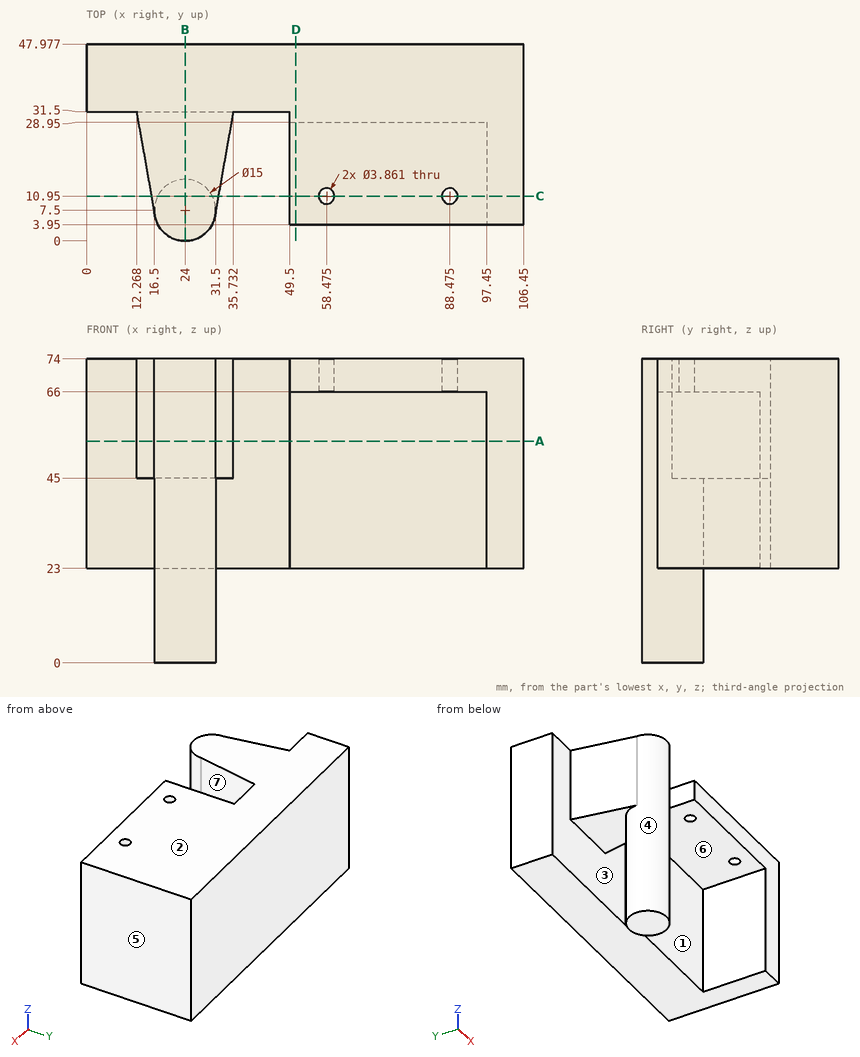
Answer from the drawing. Dimensions are ordinates in mm from the lowest x, y and z of the part. A direction names the side the tool comes from. Coordinates: 2 decimals unless noted, no trailing zeros. Write each loop counter-clockwise with the first axis right and the second up, starting at its lowest first coordinate (ties: lowest second). Pieces come first, ordered by that corner, then holes. Notation, with made-up numbers: M -13,-17 L -9,-17 A20 cw -9,6 Z; hole C 86.25,-30.75 d5. An arc over 180 degrees is marked long. Put each result on its own line as item: value. Start each with the question number.
1. A cutting plane is placed at D-D on x = 51. Write down the section's boundary in (y, z), then the cut area to 3 significant figures.
2. A cutting plane is placed at C-C on y = 10.95. Count the separate pieces of the cut face and the enclosed holes in it, then the cut area to 3 significant figures.
3. Consider line 1 (X direction, y = 18, z = 30); line 2 (Z direction, x = 26, y = 26); line 3 (Z direction, x = 52, y = 34). Determine where each line is inside the solid, lowest interval first. Write a range as from..to.
4. A cutting plane is placed at A-A on z = 54. Write down the section's boundary in (x, y).
5. Flat-ended cylindrical pins translate along their axes: P1, Ø20, axis at y = 21, z = 48, coming from the -X side; P2, Ø6, axis at x = 58.475, y = 10.95, coming from the -Z side; P3, Ø5, axis at x = 59, z = 21, coming from the +Y side; P4, Ø8.5, axis at y = 22, z = 44.5, coming from the -X side. Find the tip coordinate at first contact, or state that the pin passes through.
6. For a pull along Y with two mould halves and no side action, classify the marked faces 1, 2, 3 and 4 as pulls with the +Y half, pulls with the -Y half, needs draft (parallel to the pull), parting line crosses it, or undercut.
7. Which of the six approach directions +Z, -Z, +X, -X, +Y, -Y give full straight-line access (tool end or side, diameter ignored) to the marked faces 5, 6 and 7?
8. A cutting plane is placed at B-B on x = 24. Write down the section's boundary in (y, z), then the cut area to 3 significant figures.
Resolved:
1. outline: M 3.95,66 L 28.95,66 L 28.95,23 L 47.98,23 L 47.98,74 L 3.95,74 Z
1. area: 1,170 mm2
2. separate pieces: 4
2. enclosed holes: 0
2. area: 1,850 mm2
3. line 1: x = 97.45..106.45
3. line 2: z = 45..74
3. line 3: z = 23..74
4. outline: M 0,31.5 L 12.27,31.5 L 16.5,7.5 A7.5 ccw 31.5,7.5 L 35.73,31.5 L 49.5,31.5 L 49.5,28.95 L 97.45,28.95 L 97.45,3.95 L 106.45,3.95 L 106.45,47.98 L 0,47.98 Z
5. P1: stops at x = 12.36
5. P2: stops at z = 66
5. P3: stops at y = 47.98
5. P4: stops at x = 13.2
6. face 1: pulls with the -Y half
6. face 2: needs draft
6. face 3: undercut
6. face 4: undercut
7. face 5: +Z, -Z, +X, +Y, -Y
7. face 6: -Z, -Y
7. face 7: +Z, -Z, -Y
8. outline: M 0,0 L 15,0 L 15,45 L 31.5,45 L 31.5,23 L 47.98,23 L 47.98,74 L 0,74 Z
8. area: 2,430 mm2
